from build123d import *

# Parameters (mm, degrees)
BOSS_EXTRUDE1_DEPTH     = 4
CHAMFER1_SIZE           = 3
FILLET1_R               = 3
FILLET2_R               = 0.5
CHAMFER2_SIZE           = 0.5
BOSS_EXTRUDE2_DEPTH     = 4
FILLET3_R               = 3
FILLET4_R               = 1
CUT_EXTRUDE_THIN1_START = 0.5
SKETCH3_W               = 1.5
SKETCH3_H               = 51.000458502
CUT_EXTRUDE_THIN1_DEPTH = 44.307105588
FILLET5_R               = 0.5
SKETCH4_R               = 3
CUT_EXTRUDE1_DEPTH      = 2.5
FILLET6_R               = 0.2


with BuildPart() as part:
    # Sketch1 → Boss-Extrude1 (new body)
    with BuildSketch(Plane.XY):
        with BuildLine():
            Line((11, 11), (-11, 11))
            Line((-11, 11), (-11, 10))
            Line((-11, 10), (-21.75, 10))
            Line((-21.75, 10), (-21.75, 11))
            Line((-21.75, 11), (-21.75, 25))
            Line((-21.75, 25), (-35.75, 25))
            Line((-35.75, 25), (-35.75, -25))
            ThreePointArc((-35.75, -25), (0, -22), (35.75, -25))
            Line((35.75, -25), (35.75, 25))
            Line((35.75, 25), (21.75, 25))
            Line((21.75, 25), (21.75, 11))
            Line((21.75, 11), (21.75, 10))
            Line((21.75, 10), (11, 10))
            Line((11, 10), (11, 11))
        make_face()
        with BuildLine():
            ThreePointArc((-29.75, 16.4), (-32.25, 18.9), (-29.75, 21.4))
            Line((-29.75, 21.4), (-27.75, 21.4))
            ThreePointArc((-27.75, 21.4), (-25.25, 18.9), (-27.75, 16.4))
            Line((-27.75, 16.4), (-29.75, 16.4))
        make_face(mode=Mode.SUBTRACT)
        with BuildLine():
            Line((27.75, 21.4), (29.75, 21.4))
            ThreePointArc((29.75, 21.4), (32.25, 18.9), (29.75, 16.4))
            Line((29.75, 16.4), (27.75, 16.4))
            ThreePointArc((27.75, 16.4), (25.25, 18.9), (27.75, 21.4))
        make_face(mode=Mode.SUBTRACT)
    extrude(amount=BOSS_EXTRUDE1_DEPTH)

    # Chamfer1
    chamfer1_edges = [part.edges().sort_by_distance(p)[0] for p in [
        (-35.75, 25, 2),
        (-21.75, 25, 2),
        (21.75, 25, 2),
        (35.75, 25, 2),
    ]]
    chamfer(chamfer1_edges, length=CHAMFER1_SIZE)

    # Fillet1
    fillet1_edges = [part.edges().sort_by_distance(p)[0] for p in [
        (-21.75, 10, 2),
        (21.75, 10, 2),
        (35.75, -25, 2),
        (-35.75, -25, 2),
    ]]
    fillet(fillet1_edges, radius=FILLET1_R)

    # Fillet2
    fillet2_edges = [part.edges().sort_by_distance(p)[0] for p in [
        (-11, 10, 2),
        (11, 10, 2),
    ]]
    fillet(fillet2_edges, radius=FILLET2_R)

    # Chamfer2
    chamfer2_edges = [part.edges().sort_by_distance(p)[0] for p in [
        (-11, 11, 2),
        (11, 11, 2),
    ]]
    chamfer(chamfer2_edges, length=CHAMFER2_SIZE - 0.0001)  # a hair under: the kernel refuses the full size

    # Sketch2 → Boss-Extrude2 (add)
    with BuildSketch(Plane.XY.offset(4)):
        with BuildLine():
            Line((-0.9, -21.001879268), (-0.9, 8.998120732))
            ThreePointArc((-0.9, 8.998120732), (-17.880609494, 8.256953983), (-34.75, 6.179915017))
            Line((-34.75, 6.179915017), (-34.75, -21.479677333))
            ThreePointArc((-34.75, -21.479677333), (-34.053405155, -22.996626575), (-32.448864997, -23.456876794))
            ThreePointArc((-32.448864997, -23.456876794), (-16.719552995, -21.649540192), (-0.9, -21.001879268))
        make_face()
        with BuildLine():
            ThreePointArc((34.75, 6.179915017), (17.880609494, 8.256953983), (0.9, 8.998120732))
            Line((0.9, 8.998120732), (0.9, -21.001879268))
            ThreePointArc((0.9, -21.001879268), (16.719552995, -21.649540192), (32.448864997, -23.456876794))
            ThreePointArc((32.448864997, -23.456876794), (34.053405155, -22.996626575), (34.75, -21.479677333))
            Line((34.75, -21.479677333), (34.75, 6.179915017))
        make_face()
    extrude(amount=BOSS_EXTRUDE2_DEPTH)

    # Fillet3
    fillet3_edges = [part.edges().sort_by_distance(p)[0] for p in [
        (-0.9, -21.001879268, 6),
        (-34.75, 6.179915017, 6),
        (0.9, -21.001879268, 6),
        (34.75, 6.179915017, 6),
    ]]
    fillet(fillet3_edges, radius=FILLET3_R)

    # Fillet4
    fillet4_edges = [part.edges().sort_by_distance(p)[0] for p in [
        (-0.9, 8.998120732, 6),
        (0.9, 8.998120732, 6),
    ]]
    fillet(fillet4_edges, radius=FILLET4_R)

    # Sketch3 → Cut-Extrude-Thin1 (cut, through all)
    with BuildSketch(Plane.XY.offset(4).offset(CUT_EXTRUDE_THIN1_START)):
        with Locations((-19, -9.490221292)):
            Rectangle(SKETCH3_W, SKETCH3_H)
        with Locations((19, -9.490221292)):
            Rectangle(SKETCH3_W, SKETCH3_H)
    extrude(amount=CUT_EXTRUDE_THIN1_DEPTH, mode=Mode.SUBTRACT)

    # Fillet5
    fillet5_edges = [part.edges().sort_by_distance(p)[0] for p in [
        (-18.25, -6.7741198, 8),
        (-19.75, -6.906881766, 8),
        (19.75, -6.906881766, 8),
        (18.25, -6.7741198, 8),
    ]]
    fillet(fillet5_edges, radius=FILLET5_R)

    # Sketch4 → Cut-Extrude1 (cut)
    with BuildSketch(Plane(origin=(0, 0, 0), x_dir=(-1, 0, 0), z_dir=(0, 0, -1))):
        with Locations((-16.25, 0.5)):
            Circle(SKETCH4_R)
        with Locations((24.252501254, 0.5)):
            Circle(SKETCH4_R)
        with Locations((15.75, -13.5)):
            Circle(SKETCH4_R)
        with Locations((-25.25, -13.5)):
            Circle(SKETCH4_R)
    extrude(amount=-CUT_EXTRUDE1_DEPTH, mode=Mode.SUBTRACT)

    # Fillet6
    fillet6_edges = [part.edges().sort_by_distance(p)[0] for p in [
        (19.25, 0.5, 0),
        (-21.252501254, 0.5, 0),
        (-12.75, -13.5, 0),
        (28.25, -13.5, 0),
    ]]
    fillet(fillet6_edges, radius=FILLET6_R)


solid = part.part
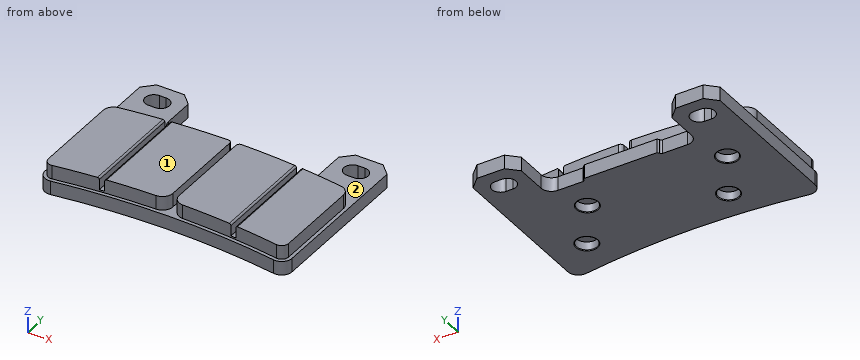
Source: CAD feature listing. Evaluate the final solid. Frame: model axes, mm. Face numbers are marked on the shaded views. Give positions to 0.01 mm unless a question says otherwise; leave off trailing zeros. Write each loop counter-clockwise with the first axis right and the second up, starting at its lowest first coordinate (ties: lowest second). Pieces come first, ordered by that corner, then holes. Notation, with made-up numbers: M 19.5,-10.75 L 24.5,-10.75 A12 cw 24.5,11.25 Z; hole C 32,89 d4. An arc over 180 degrees is marked long. Return JSON: item names as keys, results as strings. Group by question number.
1) Pull-direction query (X, two-part tool) for the marked faces 1 and 2; classes: pulls with the +X half, pulls with the -X half, needs draft (parallel to the pull), parting line crosses it, or undercut.
2) Cut plane B-B, the plane z = 5.5. Output: boundary loops of the cut face in (x, y), plus the area to 3 significant figures.
3) Material intervals for line 1 along X through (y, z) = (-18, 7.25); line 2 along X through (y, z) = (-19, 6); line 3 along Y through (x, z) = (26, 2), sorted ascending. Write a range as [from, to].
4) Cut plane D-D, the plane y = -7. Output: boundary loops of the cut face in (x, z), plus the area to 3 significant figures.
5) Cut plane C-C, the plane x = 31. Output: boundary loops of the cut face in (y, z).
6) Pin query (flat end, axial travel): P1, Ø3, axis at x = 26, y = -14, coming from the -Z side; P2, Ø1.2, axis at x = -15.5, z = 2, coming from the +Y side; P3, Ø0.6, axis at x = -29, z = 2, coming from the -Y side; P4, Ø3.5, axis at y = -13.5, z = 5.5, coming from the -X side. Return the tip coordinate at first contact, or that it passes through.
7) Cut plane A-A, the plane y = 18.9. Output: boundary loops of the cut face in (x, z).
Recorded:
{
 "1": {"face 1": "needs draft", "face 2": "undercut"},
 "2": {"outline": "M -34.75,-21.48 A2 ccw -32.45,-23.46 A215.51 cw -19.75,-21.91 L -19.75,8.09 A215.51 ccw -32.2,6.58 A3 ccw -34.75,3.61 Z; M -18.25,-21.77 A215.51 cw -3.85,-21.03 A3 ccw -0.9,-18.03 L -0.9,7.99 A1 ccw -1.91,8.99 A215.51 ccw -18.25,8.23 Z; M 0.9,-18.03 A3 ccw 3.85,-21.03 A215.51 cw 18.25,-21.77 L 18.25,8.23 A215.51 ccw 1.91,8.99 A1 ccw 0.9,7.99 Z; M 19.75,-21.91 A215.51 cw 32.45,-23.46 A2 ccw 34.75,-21.48 L 34.75,3.61 A3 ccw 32.2,6.58 A215.51 ccw 19.75,8.09 Z", "area": "1,930 mm²"},
 "3": {"line 1": "x = [-34.75, -19.75], [-18.25, -0.9], [0.9, 18.25], [19.75, 34.75]", "line 2": "x = [-34.75, -19.75], [-18.25, -1.06], [1.06, 18.25], [19.75, 34.75]", "line 3": "y = [-23.58, -16.4], [-10.6, 17.11], [20.69, 25]"},
 "4": {"outline": "M -35.75,0 L 35.75,0 L 35.75,4 L 34.75,4 L 34.75,8 L 20.25,8 A0.5 ccw 19.75,7.5 L 19.75,4.5 L 18.25,4.5 L 18.25,7.5 A0.5 ccw 17.75,8 L 0.9,8 L 0.9,4 L -0.9,4 L -0.9,8 L -17.75,8 A0.5 ccw -18.25,7.5 L -18.25,4.5 L -19.75,4.5 L -19.75,7.5 A0.5 ccw -20.25,8 L -34.75,8 L -34.75,4 L -35.75,4 Z", "area": "546 mm²"},
 "5": {"outline": "M -24.25,0 L 16.73,0 L 16.73,4 L 6.76,4 L 6.76,8 L -23.24,8 L -23.24,4 L -24.25,4 Z; M 21.07,0 L 25,0 L 25,4 L 21.07,4 Z"},
 "6": {"P1": "stops at z = 2.5", "P2": "stops at y = 10", "P3": "stops at y = -24.01", "P4": "stops at x = -35.75"},
 "7": {"outline": "M -35.75,0 L -32.25,0 L -32.25,4 L -35.75,4 Z; M -25.25,0 L -21.75,0 L -21.75,4 L -25.25,4 Z; M 21.75,0 L 25.25,0 L 25.25,4 L 21.75,4 Z; M 32.25,0 L 35.75,0 L 35.75,4 L 32.25,4 Z"}
}
